Answer from the drawing. Dimensions are ordinates in mm from the lowest x, y and z of the part. Round coordinates to 2 decimals unless told otherwise and drop trailing zeros. Loops run counter-clockwise (first coordinate to the right, second up) from the corner with the lowest first, then second, coordinate; pieces in that order, holes last. Notation, with made-up numbers: (-0.75, 17.25) - (50.25, 17.25) arc R23 ccw to (50.25, 28.25) - close; hole circle Ø8 at (27, 6.25). An arc over 180 degrees is marked (long way). Answer as CSV lines item,"result".
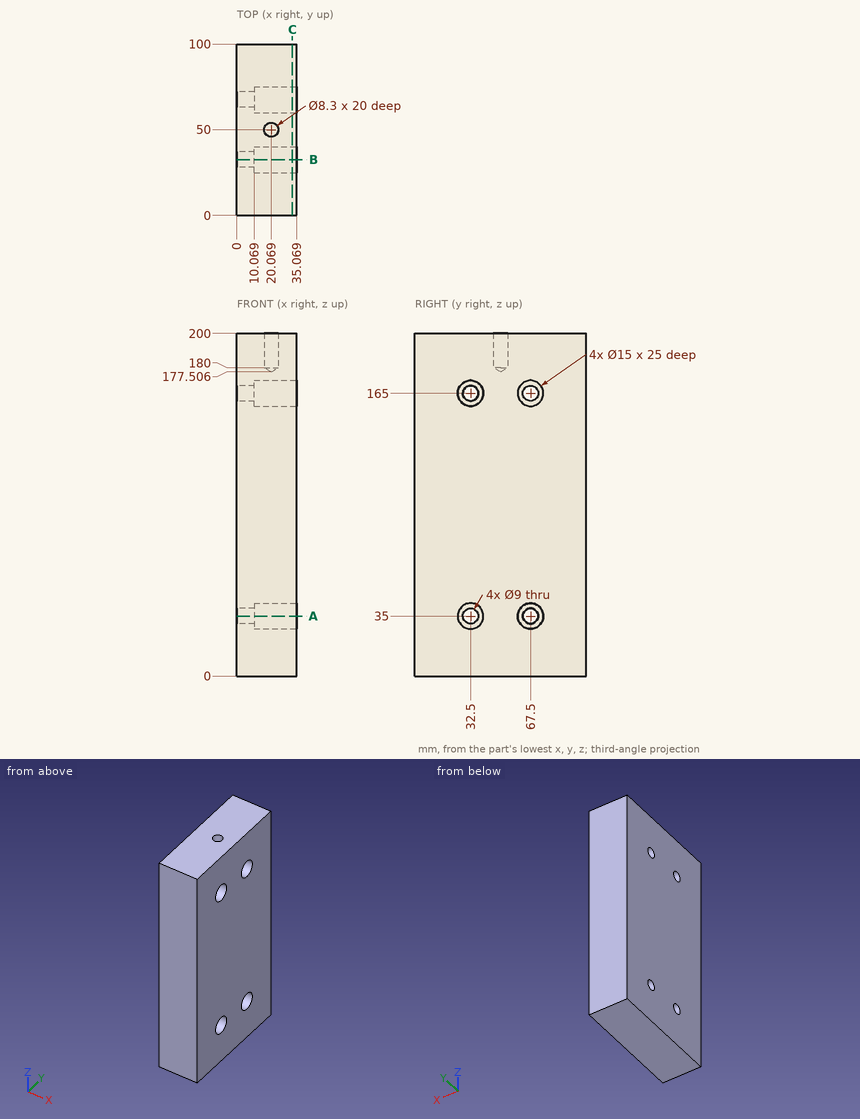
1) A cutting plane is placed at A-A, the plane z = 35. Determine the outline of the cut face in (x, y).
Entries:
outline,"(0, 0) - (35.07, 0) - (35.07, 25) - (10.07, 25) - (10.07, 28) - (0, 28) - close; (0, 37) - (10.07, 37) - (10.07, 40) - (35.07, 40) - (35.07, 60) - (10.07, 60) - (10.07, 63) - (0, 63) - close; (0, 72) - (10.07, 72) - (10.07, 75) - (35.07, 75) - (35.07, 100) - (0, 100) - close"
2) Find the intervals of material crossed by line 1 (Y direction, x = 4.5, z = 35); line 2 (Z direction, x = 29, y = 32); line 3 (Z direction, x = 4.25, y = 32.5), in increasing order.
Entries:
line 1,"y = 0 to 28, 37 to 63, 72 to 100"
line 2,"z = 0 to 27.52, 42.48 to 157.52, 172.48 to 200"
line 3,"z = 0 to 30.5, 39.5 to 160.5, 169.5 to 200"
3) A cutting plane is placed at B-B, the plane y = 32.5. Determine the outline of the cut face in (x, z).
Entries:
outline,"(0, 0) - (35.07, 0) - (35.07, 27.5) - (10.07, 27.5) - (10.07, 30.5) - (0, 30.5) - close; (0, 39.5) - (10.07, 39.5) - (10.07, 42.5) - (35.07, 42.5) - (35.07, 157.5) - (10.07, 157.5) - (10.07, 160.5) - (0, 160.5) - close; (0, 169.5) - (10.07, 169.5) - (10.07, 172.5) - (35.07, 172.5) - (35.07, 200) - (0, 200) - close"
4) Each of these flat-tipped pins is pushed along its axis until it touches: P1, Ø4.5, axis at y = 33.5, z = 38, coming from the +X side; P2, Ø8, axis at y = 67.5, z = 35, coming from the -X side. Where does it stop, or does it pass through?
Entries:
P1,"stops at x = 10.07"
P2,"passes through"
5) A cutting plane is placed at C-C, the plane x = 32.5. Determine the outline of the cut face in (y, z).
Entries:
outline,"(0, 0) - (100, 0) - (100, 200) - (0, 200) - close; hole circle Ø15 at (32.5, 35); hole circle Ø15 at (32.5, 165); hole circle Ø15 at (67.5, 35); hole circle Ø15 at (67.5, 165)"
